Autodesk Inventor part; units mm, degrees
ref_plane "YZ Plane" through (0, 0, 0) normal (1, 0, 0) x (0, 1, 0)
ref_plane "XZ Plane" through (0, 0, 0) normal (0, 1, 0) x (-1, 0, 0)
ref_plane "XY Plane" through (0, 0, 0) normal (0, 0, 1) x (1, 0, 0)
sketch "Sketch1" plane through (0, 0, 0) normal (0, 0, 1) x (1, 0, 0)
  line L0 (-490, 43) -> (490, 43)
  line L1 (490, 43) -> (490, 0)
  line L2 (490, 0) -> (-490, 0)
  line L3 (-490, 0) -> (-490, 43)
  point P0 (0, 0)
  point P1 (0, 0)
  dimension "d0" = 980
  dimension "d1" = 43
extrude "Plate1" add sketch "Sketch1" along normal blind 2
sketch "Sketch2" plane through (490, 2, 0) normal (0, -1, 0) x (1, 0, 0)
  line L0 (-980, 0) -> (0, 0)
  line L1 (0, 0) -> (0, 20)
  line L2 (0, 20) -> (-980, 20)
  line L3 (-980, 20) -> (-980, 0)
edge flange "Flange1" height 20 angle 90 thickness 2 bend radius 2.75 thickness toward (0, -1, 0) relief round relief width 2 relief depth 1 edges at (0, 0, 2) wall of the first edge with corners at (-490, 2, 0) (490, 2, 0) (490, 2, 20) (-490, 2, 20)
bend "Bend1"
corner "Corner1"
sketch "Sketch5" plane through (0, 0, 0) normal (0, 0, -1) x (-1, 0, 0)
  line L0 (490, 43) -> (-490, 43)
  line L1 (490, 0) -> (-490, 0)
  circle A0 centre (0, 43) radius 35
  line L2 (243.95, 43) -> (246.05, 43)
  line L3 (246.05, 43) -> (246.05, 29)
  line L4 (246.05, 29) -> (243.95, 29)
  line L5 (243.95, 29) -> (243.95, 43)
  line L6 (-243.95, 43) -> (-246.05, 43)
  line L7 (-246.05, 43) -> (-246.05, 29)
  line L8 (-246.05, 29) -> (-243.95, 29)
  line L9 (-243.95, 29) -> (-243.95, 43)
  line L10 (0, 43) -> (0, 0) construction
  point P0 (0, 0)
  point P1 (245, 29)
  point P2 (-245, 29)
  point P3 (246.05, 43)
  point P4 (-35, 43)
  point P5 (35, 43)
  point P6 (-246.05, 43)
  dimension "d45" = 70
  dimension "d48" = 2.1
  dimension "d49" = 490
  dimension "d51" = 29
  dimension "d52" = 14
extrude "Extrusion1" cut sketch "Sketch5" against normal through all contours L3 L4 L5 L0 | L9 L8 L7 L0 | A0 L0 picked at (-5.9248, 24.8306)
sketch "Sketch9" plane through (0, 0, 2) normal (0, 0, 1) x (1, 0, 0)
  line L0 (485.6141, 29.596) -> (485.6141, 17.596) construction
  line L1 (485.6141, 17.596) -> (285.6141, 17.596) construction
  line L2 (285.6141, 17.596) -> (285.6141, 29.596) construction
  line L3 (285.6141, 29.596) -> (485.6141, 29.596) construction
  line L4 (-490, 43) -> (490, 43)
  point P0 (0, 0)
  point P1 (1.05, 68)
  point P2 (490, 43)
  dimension "d40" = 200
  dimension "d41" = 12
mark "Mark2"
equation "\"d2\" = Thickness"
equation "\"d3\" = BendReliefWidth"
equation "\"d4\" = BendReliefDepth"
equation "\"d5\" = MinimumRemnant"
equation "\"d6\" = TransitionRadius"
equation "\"d9\" = BendRadius"
equation "\"d10\" = CornerReliefSize"
equation "\"d11\" = GapSize"
equation "\"d12\" = JacobiRadiusSize"
equation "\"BendReliefWidth\" = Thickness"
equation "\"BendReliefDepth\" = 0.5 * Thickness"
equation "\"CornerReliefSize\" = 4 * Thickness"
equation "\"MinimumRemnant\" = 2 * Thickness"
equation "\"TransitionRadius\" = BendRadius"
equation "\"JacobiRadiusSize\" = BendRadius"
equation "\"GapSize\" = Thickness"
properties part number "MSC 308 stringer BOARD  ###" material "Stainless Steel"
Design review of the part built by this model. Coordinates are the model's own, in mm. A direction names the side the tool comes from. Coordinates: 2 decimals unless noted, no trailing zeros. Write each loop counter-clockwise with the first axis right and the second up, starting at its lowest first coordinate (ties: lowest second). Pieces come first, ordered by that corner, then holes. Notation, with made-up numbers: (-8, 30.25) -> (51, 30.25) arc R22 cw to (51, 36.25) -> close; hole circle Ø1 at (79.25, -30). An arc over 180 degrees is marked (long way). Write each question's results on one line, items separated by ' | '. Start each with the question number.
(1) For line 1 along Z through (x, y) = (322, 11); line 2 along X through (y, z) = (20.5, 1), list the stretches that pass through material, from the lowest coordinate up. Write a range as from..to.
(2) Clearance check with flat-ended pins moving along their axes: P1, Ø1, axis at x = -245.5, z = 1.5, coming from the +Y side; P2, Ø2, axis at x = 84, z = 15, coming from the +Y side; P3, Ø6, axis at x = -101.5, y = 36.5, coming from the +Z side. State where each tip first meets the part, or that it passes through.
(3) Take a section at B-B on y = 15.5. Write out the cut boundary in (x, z).
(4) Take a section at C-C on x = 0. Write out the cut boundary in (y, z).
(5) The part is to be moulded in two halves that separate along X. For faces 1 (the face through (0.77, 8.01, 0.99)), 2 (the face through (490, 17, 1)), 3 (the face through (-490, 17, 1)), 4 (the face through (-7, 7, 2)), say which applies: pulls with the +X half, pulls with the -X half, needs draft (parallel to the pull), parting line crosses it, or undercut.
(6) Take a section at A-A on x = -201.5. Write out the cut boundary in (y, z), and give its area (3 significant figures).
(7) Tool access review of faces 5 (the face through (-7, 7, 0)), 6 (the face through (7, 2, 12)): name each direction out of +Z, -Z, +X, -X, +Y, -Y from which nothing blocks a thin tool from reaching the whole face with its end or side.
(8) Take a section at D-D on z = 10.75. Write out the cut boundary in (x, y), and give its area (3 significant figures).
Results found:
1) line 1: z = 0..2 | line 2: x = -490..-26.81, 26.81..490
2) P1: stops at y = 29 | P2: stops at y = 2 | P3: stops at z = 2
3) outline: (-490, 0) -> (-21.65, 0) -> (-21.65, 2) -> (-490, 2) -> close; (21.65, 0) -> (490, 0) -> (490, 2) -> (21.65, 2) -> close
4) outline: (0, 4.75) arc R4.75 ccw to (4.75, 0) -> (8, 0) -> (8, 2) -> (4.75, 2) arc R2.75 cw to (2, 4.75) -> (2, 20) -> (0, 20) -> close
5) face 1: undercut | face 2: pulls with the +X half | face 3: pulls with the -X half | face 4: needs draft
6) outline: (0, 4.75) arc R4.75 ccw to (4.75, 0) -> (43, 0) -> (43, 2) -> (4.75, 2) arc R2.75 cw to (2, 4.75) -> (2, 20) -> (0, 20) -> close | area: 119 mm2
7) face 5: -Z, +X, -X, +Y, -Y | face 6: +Z, +X, -X, +Y
8) outline: (-490, 0) -> (490, 0) -> (490, 2) -> (-490, 2) -> close | area: 1,960 mm2
